Verification items for this drawing (mm, ordinates from the low corner). A direction names the side the tool comes from. Coordinates: 2 decimals unless noted, no trailing zeros. Loops run counter-clockwise (first coordinate to the right, second up) from the corner with the lowest first, then second, coordinate; pieces in that order, holes last. Notation, with made-up numbers: (84, -32) - (126, -32) arc R17 cw to (126, -13) - close; hole circle Ø10 at (68, 47). An arc over 180 degrees is marked (long way). Write each question's results on one line, items separated by ' | '. Start each with the question number.
(1) Go/stop test with flat-tipped pins: pin 1 Ø1.5 at (y, z) = (3.5, 20.5) entering from +X; pin 2 Ø4 at (x, z) = (50, 28) entering from +Y; pin 3 Ø1.6 at (x, z) = (56, 8.5) entering from +Y; pin 4 Ø1 at (x, z) = (22, 21.5) entering from -Y. Record where each tip stops, or that it passes through.
(2) Sectioned sample at D-D (z = 9). Enter the section's corners in (x, y), plus the area to 3 significant figures.
(3) Access from +Z, -Z, +X, -X, +Y, -Y to the whole of each face (thin tool, end or side, straight path). Record for the marked faces 4 and 5.
(4) Sectioned sample at B-B (x = 38.7). Enter the section's corners in (y, z), plus the area to 3 significant figures.
(5) Mould release check, pull along Z, two halves, no side actions. Record for the marked faces 1, 2 and 3: pulls with the +Z half, pulls with the -Z half, needs draft (parallel to the pull), parting line crosses it, or undercut.
(6) Sectioned sample at A-A (x = 45). Enter the section's corners in (y, z), plus the area to 3 significant figures.
(7) Material ranges on probe 1 along X at (y, z) = (1.55, 4.7); probe 2 along Z at (x, y) = (13, 1.5); probe 3 along Z at (x, y) = (44, 4), recorded low to high.
(8) Sectioned sample at C-C (y = 10). Enter the section's corners in (x, z), plus the area to 3 significant figures.
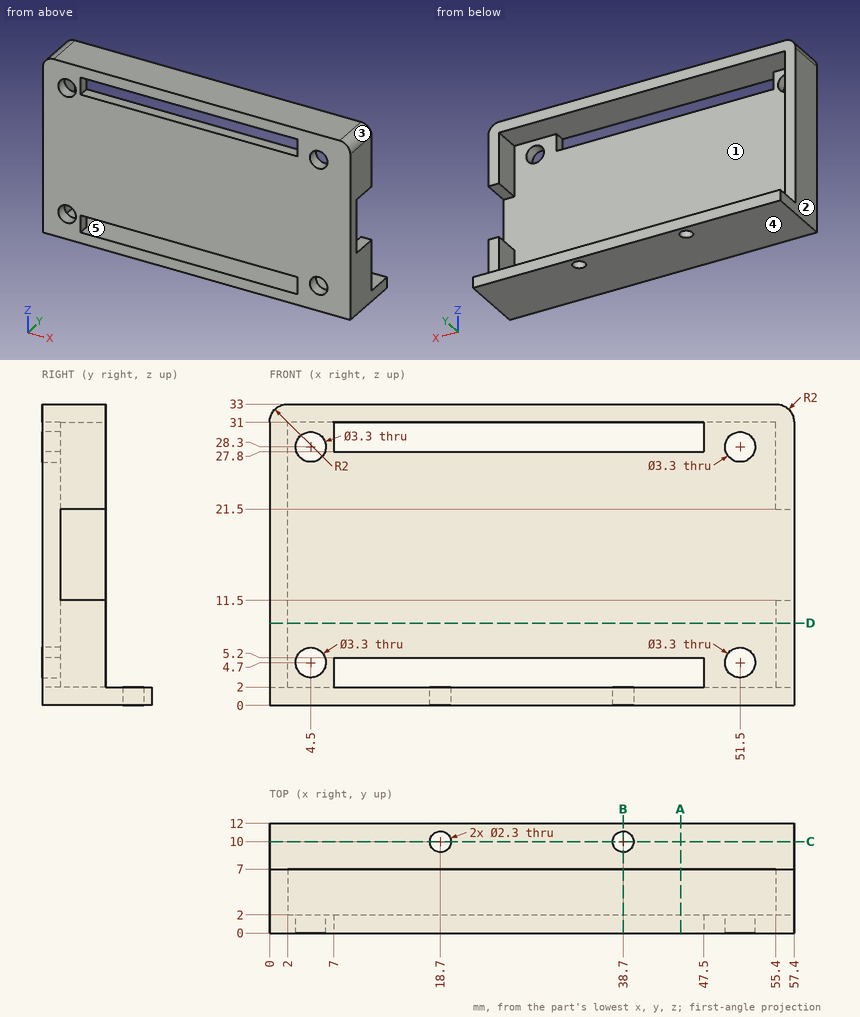
Outcome:
1) pin 1: stops at x = 2 | pin 2: stops at y = 2 | pin 3: stops at y = 7 | pin 4: stops at y = 0
2) outline: (0, 0) - (57.4, 0) - (57.4, 7) - (55.4, 7) - (55.4, 2) - (2, 2) - (2, 7) - (0, 7) - close | area: 135 mm2
3) face 4: -Z, +X, -X, +Y, -Y | face 5: +Y
4) outline: (0, 0) - (8.85, 0) - (8.85, 2) - (0, 2) - close; (0, 5.2) - (2, 5.2) - (2, 27.8) - (0, 27.8) - close; (0, 31) - (7, 31) - (7, 33) - (0, 33) - close; (11.15, 0) - (12, 0) - (12, 2) - (11.15, 2) - close | area: 78.6 mm2
5) face 1: undercut | face 2: needs draft | face 3: pulls with the +Z half
6) outline: (0, 0) - (12, 0) - (12, 2) - (0, 2) - close; (0, 5.2) - (2, 5.2) - (2, 27.8) - (0, 27.8) - close; (0, 31) - (7, 31) - (7, 33) - (0, 33) - close | area: 83.2 mm2
7) probe 1: x = 0 to 2.85, 6.15 to 7, 47.5 to 49.85, 53.15 to 57.4 | probe 2: z = 0 to 2, 5.2 to 27.8, 31 to 33 | probe 3: z = 0 to 2, 31 to 33
8) outline: (0, 0) - (17.55, 0) - (17.55, 2) - (0, 2) - close; (19.85, 0) - (37.55, 0) - (37.55, 2) - (19.85, 2) - close; (39.85, 0) - (57.4, 0) - (57.4, 2) - (39.85, 2) - close | area: 106 mm2
